Geometry: final body of the model. Coordinates: model frame, mm. A direction names the side the tool comes from. Give positions to 0.01 mm unless a question says otherwise; leave off trailing zeros. Order: outer loops, then holes, each group sorted by start corner. A loop starts at its lowest first (then second) coordinate and runs counter-clockwise, first axis right, second up. Notation, with made-up numbers: (-7.75, -14.5) -> (51.25, -14.5) arc R29 ccw to (51.25, 15.5) -> close; hole circle Ø6 at (-28.5, 81). An arc over 180 degrees is marked (long way). Answer in a Markdown table with one row per item. Add a question column.
Q1. Line query: line 1 along Z through (x, y) = (64.25, 4); line 2 along X through (y, z) = (13.5, 5.5) (3 decimals); line 3 along X through (y, z) = (4.25, -10.5) (3 decimals). Output: solid intervals per line, ascending. Write a range as from..to.
Q2. Contact query for flat-ended pins moving along their axis: P1, Ø6, axis at y = 9.5, z = 15, coming from the -X side; P2, Ø3.5, axis at x = 0, z = 0, coming from the +Y side; P3, Ø5, axis at y = 4.5, z = 18.5, coming from the -X side (3 decimals); P4, Ø1.8, axis at y = 4, z = 0, coming from the +X side (3 decimals). Output: stop coordinate, or through.
Q3. Cut plane A-A on y = 8.5. Return the cut outline in (x, z) (3 decimals).
Q4. Pull-direction query (X, two-part tool) for faces 6 (the face through (70.775, 12, 2)), 7 (the face through (44.887, 8.112, 0.105)), 8 (the face through (-16, 16, 30)); classes: +X half, -X half, draft (parallel to the pull), parting line (faces both ways), or undercut.
Q5. Cut plane B-B on z = 0. Count the separate pieces of the cut face and the enclosed holes in it, and give its area (3 significant figures).
Q6. Set-up query: faces 1 (the face through (33.775, 6, -8)), 2 (the face through (-33.775, 6, 0)), 3 (the face through (-16.651, 5.817, -29.386)), 4 (the face through (65.7, 2.57, 0.45)), 5 (the face through (0, 14, 8)). Return all of +Z, -Z, +X, -X, +Y, -Y with unobstructed straight access to the full face (end or side cutting, diameter ignored); none if empty.
from build123d import *

# Parameters (mm, degrees)
BOSS_EXTRUDE1_DEPTH      = 14
BOSS_EXTRUDE2_DEPTH      = 2
BOSS_EXTRUDE2_DEPTH_BACK = 0.2
CHAMFER1_SIZE            = 2
SKETCH3_R                = 2
CUT_EXTRUDE1_DEPTH       = 57.412025139
BOSS_EXTRUDE3_DEPTH      = 7.5
CUT_EXTRUDE2_REACH       = 110.187
SKETCH6_R                = 1.5
CHAMFER2_SIZE            = 1
CHAMFER3_SIZE            = 3


with BuildPart() as part:
    # Sketch1 → Boss-Extrude1 (new body)
    with BuildSketch(Plane(origin=(0, 0, 0), x_dir=(1, 0, 0), z_dir=(0, 1, 0))):
        Polygon((33.774990748, 19.5), (0, 39), (-33.774990748, 19.5), (-33.774990748, -19.5), (0, -39), (33.774990748, -19.5), align=None)
    extrude(amount=BOSS_EXTRUDE1_DEPTH)

    # Sketch2 → Boss-Extrude2 (add, two sides: drawn at the far end of the back side and taken through both)
    with BuildSketch(Plane(origin=(0, 14, 0), x_dir=(1, 0, 0), z_dir=(0, 1, 0)).offset(-BOSS_EXTRUDE2_DEPTH_BACK)):
        Polygon((0, 41.309401077), (-35.774990748, 20.654700538), (-35.774990748, -20.654700538), (0, -41.309401077), (35.774990748, -20.654700538), (35.774990748, 20.654700538), align=None)
        Polygon((33.774990748, -19.5), (33.774990748, 19.5), (0, 39), (-33.774990748, 19.5), (-33.774990748, -19.5), (0, -39), align=None, mode=Mode.SUBTRACT)
    extrude(amount=BOSS_EXTRUDE2_DEPTH + BOSS_EXTRUDE2_DEPTH_BACK)

    # Chamfer1
    chamfer1_edges = [part.edges().sort_by_distance(p)[0] for p in [
        (-16.887495374, 13.8, 29.25),
        (16.887495374, 13.8, 29.25),
        (33.774990748, 13.8, 0),
        (16.887495374, 13.8, -29.25),
        (-16.887495374, 13.8, -29.25),
        (-33.774990748, 13.8, 0),
    ]]
    chamfer(chamfer1_edges, length=CHAMFER1_SIZE - 0.0001)  # a hair under: the kernel refuses the full size

    # Sketch3 → Cut-Extrude1 (cut, through all)
    with BuildSketch(Plane(origin=(0, 14, 0), x_dir=(1, 0, 0), z_dir=(0, 1, 0))):
        with Locations(Location((0, 0, 0), (0, 0, 270))):
            Circle(SKETCH3_R)
    extrude(amount=-CUT_EXTRUDE1_DEPTH, mode=Mode.SUBTRACT)

    # Sketch5 → Boss-Extrude3 (add, symmetric)
    with BuildSketch(Plane.XY):
        Polygon((33.774990748, 11.8), (34.432855124, 11.8), (48.632855124, 26), (70.774990748, 26), (70.774990748, 0), (60.774990748, 0), (60.774990748, 16), (52.774990748, 16), (36.774990748, 0), (33.774990748, 0), align=None)
    extrude(amount=BOSS_EXTRUDE3_DEPTH, both=True)

    # Sketch6 → Cut-Extrude2 (cut, up to next)
    with BuildSketch(Plane.ZY.offset(-60.774990748), mode=Mode.PRIVATE) as cut_extrude2_sk1:
        with Locations(Location((0, 12, 0), (0, 0, 270))):
            Circle(SKETCH6_R)
    cut_extrude2_tool1 = extrude(cut_extrude2_sk1.sketch, amount=-CUT_EXTRUDE2_REACH, mode=Mode.PRIVATE) & part.part
    # Sketch6 → Cut-Extrude2 (cut, up to next)
    with BuildSketch(Plane.ZY.offset(-60.774990748), mode=Mode.PRIVATE) as cut_extrude2_sk2:
        with Locations(Location((0, 4, 0), (0, 0, 270))):
            Circle(SKETCH6_R)
    cut_extrude2_tool2 = extrude(cut_extrude2_sk2.sketch, amount=-CUT_EXTRUDE2_REACH, mode=Mode.PRIVATE) & part.part
    add(cut_extrude2_tool1.solids().sort_by_distance((60.774991, 12, 0))[0], mode=Mode.SUBTRACT)
    add(cut_extrude2_tool2.solids().sort_by_distance((60.774991, 4, 0))[0], mode=Mode.SUBTRACT)

    # Chamfer2
    chamfer2_edges = [part.edges().sort_by_distance(p)[0] for p in [
        (60.774990748, 16, 0),
    ]]
    chamfer(chamfer2_edges, length=CHAMFER2_SIZE)

    # Chamfer3
    chamfer3_edges = [part.edges().sort_by_distance(p)[0] for p in [
        (70.774990748, 26, 0),
    ]]
    chamfer(chamfer3_edges, length=CHAMFER3_SIZE)


solid = part.part
Completed:
| question | item | result |
|---|---|---|
| 1 | line 1 | z = -7.5..-1.5, 1.5..7.5 |
| 1 | line 2 | x = -35.475..35.475, 36.133..50.275, 60.775..70.775 |
| 1 | line 3 | x = -33.775..33.775 |
| 2 | P1 | stops at x = -34.47 |
| 2 | P2 | passes through |
| 2 | P3 | stops at x = -33.775 |
| 2 | P4 | stops at x = 41.675 |
| 3 | outline | (-33.775, -19.5) -> (0, -39) -> (33.775, -19.5) -> (33.775, -7.5) -> (45.275, -7.5) -> (45.275, 7.5) -> (33.775, 7.5) -> (33.775, 19.5) -> (0, 39) -> (-33.775, 19.5) -> close; (60.775, -7.5) -> (70.775, -7.5) -> (70.775, 7.5) -> (60.775, 7.5) -> close; hole circle Ø4 at (0, 0) |
| 4 | face 6 | +X half |
| 4 | face 7 | undercut |
| 4 | face 8 | draft |
| 5 | separate pieces | 4 |
| 5 | enclosed holes | 0 |
| 5 | area | 1,430 mm² |
| 6 | face 1 | +X, -Y |
| 6 | face 2 | +Z, -Z, -X, -Y |
| 6 | face 3 | -Z, -X, -Y |
| 6 | face 4 | +X |
| 6 | face 5 | +Y |
